```python
from build123d import *

# Parameters (mm, degrees)
F0_R     = 42.723605
F1_DEPTH = 40
F2_W     = 26.663388
F2_H     = 23.562994
F3_DEPTH = 40.001
F4_SIZE  = 5
F5_R     = 5
F6_R     = 5


with BuildPart() as f1:
    # F0 (on Top) → F1 (new body)
    with BuildSketch(Plane.XY):
        Circle(F0_R)
    extrude(amount=F1_DEPTH)

    # F2 (on Top) → F3 (cut, through all)
    with BuildSketch(Plane.XY):
        Rectangle(F2_W, F2_H)
    extrude(amount=F3_DEPTH, mode=Mode.SUBTRACT)

    # F4
    f4_edges = [f1.edges().sort_by_distance(p)[0] for p in [
        (0, 11.781497, 40),
        (13.331694, 0, 40),
        (-13.331694, 0, 40),
        (0, -11.781497, 40),
    ]]
    chamfer(f4_edges, length=F4_SIZE)

    # F5
    f5_edges = [f1.edges().sort_by_distance(p)[0] for p in [
        (-42.723605, 0, 40),
    ]]
    fillet(f5_edges, radius=F5_R)

    # F6
    f6_edges = [f1.edges().sort_by_distance(p)[0] for p in [
        (-42.723605, 0, 0),
    ]]
    fillet(f6_edges, radius=F6_R)


solid = f1.part
```
Source: CAD feature listing. Evaluate the final solid. Frame: model axes, mm. A direction names the side the tool comes from. Give positions to 0.01 mm unless a question says otherwise; leave off trailing zeros. Write each loop counter-clockwise with the first axis right and the second up, starting at its lowest first coordinate (ties: lowest second). Pieces come first, ordered by that corner, then holes.
1. Pull-direction query (X, two-part tool) for faces 4 (the face through (40.75, 12.83, 19.79)), 5 (the face through (-1, 17, 40)), 6 (the face through (0, 11.781, 17)); classes: +X half, -X half, draft (parallel to the pull), parting line (faces both ways), or undercut.
2. Access query for faces 1 (the face through (0, -11.781, 17)), 2 (the face through (-15.8, 0.23, 37.47)), 3 (the face through (-1, -16, 0)). Directions: +Z, -Z, +X, -X, +Y, -Y. A direction counts if a zero-diameter tool reaches every point of the face in a straight line with its end or side. Return the directions, or none.
3. Section query C-C (z = 31.5). Return the cut outline in (x, y).
4. Section query B-B (x = 0). Return the cut outline in (y, z).
5. First-contact query: pin 1 (4 mm diameter, centred on y = 19, z = 16, fed in from -X); pin 2 (3 mm diameter, centred on x = 3, z = 14.5, fed in from +Y); pin 3 (8 mm diameter, centred on x = -3.5, z = 16.5, fed in from -Y). Flat tips, straight axial feed; report the tip coordinate or a pass-through.
6. Section query A-A (y = 0). Return the cut outline in (x, z), then the cut area to 3 significant figures.
7. Material intervals for line 1 along X through (y, z) = (-8, 14); line 2 along Y through (x, z) = (7, 12); line 3 along X through (y, z) = (2, 23.5), sorted ascending.
Output values:
1. face 4: parting line
1. face 5: draft
1. face 6: undercut
2. face 1: +Z, -Z
2. face 2: +Z
2. face 3: -Z, +X, -X, +Y, -Y
3. outline: circle Ø85.45 at (0, 0); hole (-13.33, -11.78) - (13.33, -11.78) - (13.33, 11.78) - (-13.33, 11.78) - close
4. outline: (-42.72, 5) arc R5 ccw to (-37.72, 0) - (-11.78, 0) - (-11.78, 35) - (-16.78, 40) - (-37.72, 40) arc R5 ccw to (-42.72, 35) - close; (11.78, 0) - (37.72, 0) arc R5 ccw to (42.72, 5) - (42.72, 35) arc R5 ccw to (37.72, 40) - (16.78, 40) - (11.78, 35) - close
5. pin 1: stops at x = -39.2
5. pin 2: stops at y = 42.7
5. pin 3: stops at y = -42.72
6. outline: (-42.72, 5) arc R5 ccw to (-37.72, 0) - (-13.33, 0) - (-13.33, 35) - (-18.33, 40) - (-37.72, 40) arc R5 ccw to (-42.72, 35) - close; (13.33, 0) - (37.72, 0) arc R5 ccw to (42.72, 5) - (42.72, 35) arc R5 ccw to (37.72, 40) - (18.33, 40) - (13.33, 35) - close
6. area: 2,300 mm2
7. line 1: x = -41.97 to -13.33, 13.33 to 41.97
7. line 2: y = -42.15 to -11.78, 11.78 to 42.15
7. line 3: x = -42.68 to -13.33, 13.33 to 42.68
